Can you work these out from the drawing? Everything is in mm from the part's minimum corner. A direction names the side the tool comes from. Round coordinates to 2 decimals unless told otherwise and drop trailing zeros. Order: outer loops, then holes, each group sorted by start corner. A loop starts at its lowest first (then second) coordinate and runs counter-clockwise, first axis right, second up. Notation, with made-up numbers: M 4,8 L 16,8 A31 ccw 16,47 Z; hole C -13.5,20 d2. An arc over 180 degrees is marked long. Answer as CSV lines item,"result". Start each with the question number.
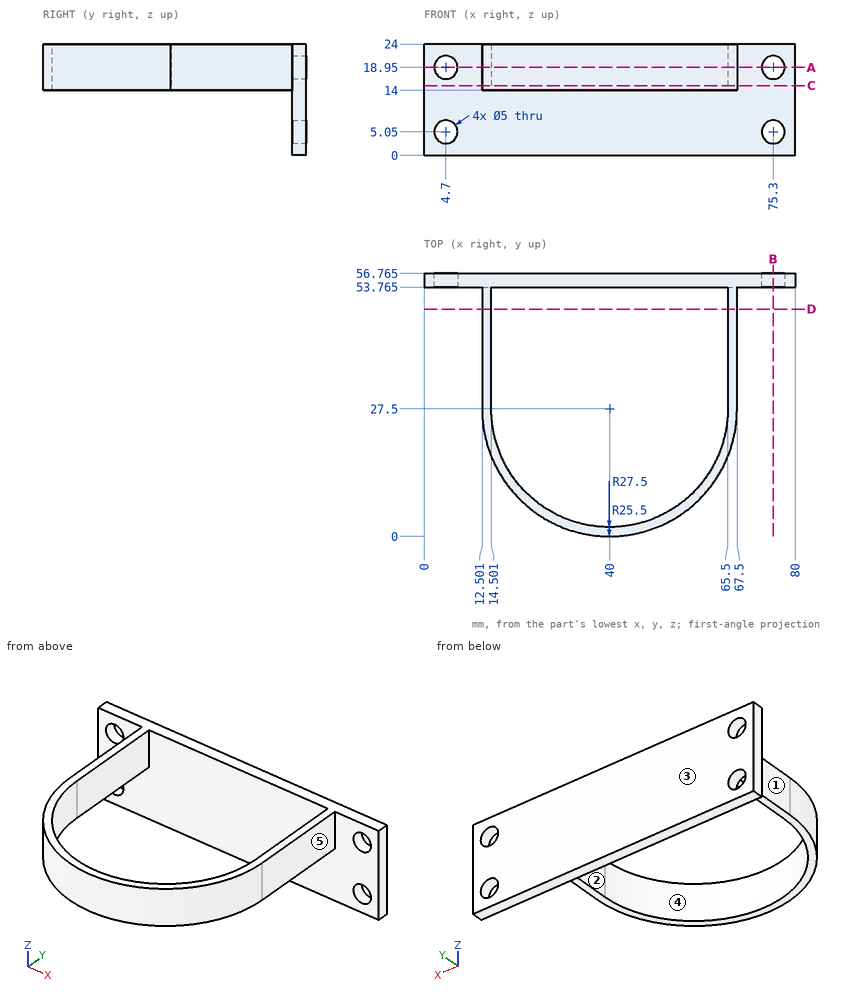
(1) If I drill on line 1 along Z through (x, y) = (4.7, 54.4); line 2 along X through (y, z) = (43.5, 17.5); line 3 along Y through (x, z) = (54.5, 8.75) (1 decimal), over which ranges is the centre line in solid material (lowest first)?
(2) I want a section at D-D on y = 49. Write out the boundary of the cut face in (x, z).
(3) If we mould it in two halves opening along X, with no side actions, what happens to the marked faces 1, 2 and 3? For each: +X half, -X half, draft (parallel to the pull), parting line (faces both ways), or undercut.
(4) For the marked faces 4 and 5, which set-ups out of +Z, -Z, +X, -X, +Y, -Y let a thin tool reach every point of the face, with its end or its side?
(5) I want a section at C-C on z = 15. Write out the boundary of the cut face in (x, y) (1 decimal).
(6) I want a section at B-B on x = 75.3. Count the separate pieces of the cut face and the enclosed holes in it, and give its area (3 significant figures).
(7) I want a section at A-A on z = 18.95. Write out the boundary of the cut face in (x, y) (1 decimal).
(8) I'm going to push flat-ended pins straight in: P1, Ø3, axis at y = 37, z = 18.5, coming from the +X side; P2, Ø12, axis at x = 34, z = 17, coming from the -Y side; P3, Ø5, axis at x = 50.5, z = 7, coming from the -Y side (1 decimal). Where does each tip first touch, or does it pass through?
From the geometry:
1,line 1,"0 to 2.55, 7.55 to 16.45, 21.45 to 24"
1,line 2,"12.5 to 14.5, 65.5 to 67.5"
1,line 3,"53.8 to 56.8"
2,outline,"M 12.5,14 L 14.5,14 L 14.5,24 L 12.5,24 Z; M 65.5,14 L 67.5,14 L 67.5,24 L 65.5,24 Z"
3,face 1,"-X half"
3,face 2,"undercut"
3,face 3,"draft"
4,face 4,"+Z, -Z"
4,face 5,"+Z, -Z, +X, -Y"
5,outline,"M 0,53.8 L 12.5,53.8 L 12.5,27.7 A27.5 ccw 67.5,27.4 L 67.5,53.8 L 80,53.8 L 80,56.8 L 0,56.8 Z; hole M 14.5,27.7 A25.5 ccw 65.5,27.4 L 65.5,53.8 L 14.5,53.8 Z"
6,separate pieces,"3"
6,enclosed holes,"0"
6,area,"42.0 mm²"
7,outline,"M 0,53.8 L 2.2,53.8 L 2.2,56.8 L 0,56.8 Z; M 7.2,53.8 L 12.5,53.8 L 12.5,27.7 A27.5 ccw 67.5,27.4 L 67.5,53.8 L 72.8,53.8 L 72.8,56.8 L 7.2,56.8 Z; M 77.8,53.8 L 80,53.8 L 80,56.8 L 77.8,56.8 Z; hole M 14.5,27.7 A25.5 ccw 65.5,27.4 L 65.5,53.8 L 14.5,53.8 Z"
8,P1,"x = 67.5"
8,P2,"y = 0"
8,P3,"y = 53.8"
